Input: part model. Units: mm. Frame: model coordinates. A direction names the side the tool comes from. Round coordinates to 2 decimals unless told otherwise and drop trailing zeros. Order: outer loops, then holes, each group sorted by start corner. A loop starts at its lowest first (then second) coordinate and runs counter-clockwise, first axis right, second up. Notation, with made-up numbers: (-4, 16) - (15, 16) arc R35 ccw to (15, 55) - close; hole circle Ø10 at (-21, 85.5). An arc over 180 degrees is marked (long way). One line per item, written item: value. Start each with the question number.
from build123d import *

# Parameters (mm, degrees)
SKETCH1_W           = 50
SKETCH1_H           = 50
BOSS_EXTRUDE1_DEPTH = 100
SKETCH2_R           = 19.9
CUT_EXTRUDE2_DEPTH  = 50
SKETCH2_5_R         = 20
SKETCH2_5_R_2       = 19.9
CUT_EXTRUDE3_DEPTH  = 40
SKETCH2_6_R         = 20.1
SKETCH2_6_R_2       = 20
CUT_EXTRUDE4_DEPTH  = 30
SKETCH2_7_R         = 20.2
SKETCH2_7_R_2       = 20.1
CUT_EXTRUDE5_DEPTH  = 20
SKETCH2_8_R         = 20.3
SKETCH2_8_R_2       = 20.2
CUT_EXTRUDE6_DEPTH  = 10


with BuildPart() as part:
    # Sketch1 → Boss-Extrude1 (new body)
    with BuildSketch(Plane(origin=(0, 0, 0), x_dir=(1, 0, 0), z_dir=(0, 1, 0))):
        Rectangle(SKETCH1_W, SKETCH1_H)
    extrude(amount=BOSS_EXTRUDE1_DEPTH)

    # Sketch2 → Cut-Extrude2 (cut)
    with BuildSketch(Plane(origin=(0, 100, 0), x_dir=(1, 0, 0), z_dir=(0, 1, 0))):
        with Locations(Location((0, 0, 0), (0, 0, 270))):
            Circle(SKETCH2_R)
    extrude(amount=-CUT_EXTRUDE2_DEPTH, mode=Mode.SUBTRACT)

    # Sketch2_5 → Cut-Extrude3 (cut)
    with BuildSketch(Plane(origin=(0, 100, 0), x_dir=(1, 0, 0), z_dir=(0, 1, 0))):
        with Locations(Location((0, 0, 0), (0, 0, 270))):
            Circle(SKETCH2_5_R)
        with Locations(Location((0, 0, 0), (0, 0, 270))):
            Circle(SKETCH2_5_R_2, mode=Mode.SUBTRACT)
    extrude(amount=-CUT_EXTRUDE3_DEPTH, mode=Mode.SUBTRACT)

    # Sketch2_6 → Cut-Extrude4 (cut)
    with BuildSketch(Plane(origin=(0, 100, 0), x_dir=(1, 0, 0), z_dir=(0, 1, 0))):
        with Locations(Location((0, 0, 0), (0, 0, 270))):
            Circle(SKETCH2_6_R)
        with Locations(Location((0, 0, 0), (0, 0, 270))):
            Circle(SKETCH2_6_R_2, mode=Mode.SUBTRACT)
    extrude(amount=-CUT_EXTRUDE4_DEPTH, mode=Mode.SUBTRACT)

    # Sketch2_7 → Cut-Extrude5 (cut)
    with BuildSketch(Plane(origin=(0, 100, 0), x_dir=(1, 0, 0), z_dir=(0, 1, 0))):
        with Locations(Location((0, 0, 0), (0, 0, 270))):
            Circle(SKETCH2_7_R)
        with Locations(Location((0, 0, 0), (0, 0, 270))):
            Circle(SKETCH2_7_R_2, mode=Mode.SUBTRACT)
    extrude(amount=-CUT_EXTRUDE5_DEPTH, mode=Mode.SUBTRACT)

    # Sketch2_8 → Cut-Extrude6 (cut)
    with BuildSketch(Plane(origin=(0, 100, 0), x_dir=(1, 0, 0), z_dir=(0, 1, 0))):
        with Locations(Location((0, 0, 0), (0, 0, 270))):
            Circle(SKETCH2_8_R)
        with Locations(Location((0, 0, 0), (0, 0, 270))):
            Circle(SKETCH2_8_R_2, mode=Mode.SUBTRACT)
    extrude(amount=-CUT_EXTRUDE6_DEPTH, mode=Mode.SUBTRACT)


solid = part.part
Item 1: Section query B-B on z = 0. Return loops of the section in (x, y), and give its area (3 significant figures).
Item 2: Pull-direction query (Z, two-part tool) for faces 3 (the face through (-11.5, 100, -17)), 4 (the face through (0, 49, 25)), 5 (the face through (-12.29, 85.07, -16.03)), 6 (the face through (0.88, 75.07, -20.08)); classes: released by +Z, released by -Z, zero draft, split by the parting line, or undercut.
Item 3: First-contact query: pin 1 Ø8 at (x, z) = (19, 15) entering from -Y; pin 2 Ø12 at (x, z) = (0, -4.5) entering from +Y. Flat tips, straight axial feed; report the tip coordinate or a pass-through.
Item 4: Section query A-A on x = 0. Return loops of the section in (y, z), and give its area (3 significant figures).
Item 5: Line query: L1, parallel to X at y = 55.5, z = 0; L2, parallel to X at y = 74.75, z = 0; L3, parallel to Y at x = 0, z = 14.5. Output: solid intervals per line, ascending.
Item 6: Reachability of faces 1 (the face through (-25, 49, 0)), 2 (the face through (-19.427, 55.07, -4.314)) from +Z, -Z, +X, -X, +Y, -Y: full face, straight path, thin tool, end or side. Return the list, or none.
Geometry results:
1. outline: (-25, 0) - (25, 0) - (25, 100) - (20.3, 100) - (20.3, 90) - (20.2, 90) - (20.2, 80) - (20.1, 80) - (20.1, 70) - (20, 70) - (20, 60) - (19.9, 60) - (19.9, 50) - (-19.9, 50) - (-19.9, 60) - (-20, 60) - (-20, 70) - (-20.1, 70) - (-20.1, 80) - (-20.2, 80) - (-20.2, 90) - (-20.3, 90) - (-20.3, 100) - (-25, 100) - close
1. area: 2,990 mm^2
2. face 3: zero draft
2. face 4: released by +Z
2. face 5: undercut
2. face 6: undercut
3. pin 1: stops at y = 0
3. pin 2: stops at y = 50
4. outline: (0, -25) - (100, -25) - (100, -20.3) - (90, -20.3) - (90, -20.2) - (80, -20.2) - (80, -20.1) - (70, -20.1) - (70, -20) - (60, -20) - (60, -19.9) - (50, -19.9) - (50, 19.9) - (60, 19.9) - (60, 20) - (70, 20) - (70, 20.1) - (80, 20.1) - (80, 20.2) - (90, 20.2) - (90, 20.3) - (100, 20.3) - (100, 25) - (0, 25) - close
4. area: 2,990 mm^2
5. L1: x = -25 to -19.9, 19.9 to 25
5. L2: x = -25 to -20.1, 20.1 to 25
5. L3: y = 0 to 50
6. face 1: +Z, -Z, -X, +Y, -Y
6. face 2: +Y
